Part model, mm, in its own coordinate system. Face numbers are marked on the shaded views. A direction names the side the tool comes from. Round coordinates to 2 decimals unless told otherwise and drop trailing zeros. Write each loop counter-clockwise with the first axis right and the second up, starting at its lowest first coordinate (ties: lowest second). Pieces come first, ordered by that corner, then holes. Notation, with made-up numbers: M 62,86 L 90,86 A22 ccw 90,105 Z; hole C 8,31 d8. An arc over 180 degrees is marked long. Use a Markdown table: item, result. Add a question column.
1) Slice it at D-D on x = 7.5. Write the cut outline in (y, z), plus the area to 3 significant figures.
2) Slice it at C-C on z = 10. Write the cut outline in (x, y), plus the area to 3 significant figures.
3) Slice it at B-B on y = 4. Write the cut outline in (x, z), plus the area to 3 significant figures.
4) Two-plate mould, pull along X, no slides. Class the marked faces 1, 2, 3 and 4: released by +X, released by -X, zero draft, split by the parting line, or undercut.
5) Which spindle directions (+Z, -Z, +X, -X, +Y, -Y) get a long thin tool onto all of the face, cutting with end or side? Do the marked faces 5 and 6. Say none if no direction does.
6) Slice it at A-A on x = 3.5. Write the cut outline in (y, z), plus the area to 3 significant figures.
7) Wall check: probe 1 along Z at (x, y) = (11.5, 6.25); probe 2 along X at (y, z) = (3.75, 9.25); probe 3 along Z at (x, y) = (7.25, 5). Give the ranges that are in metal, low to high.
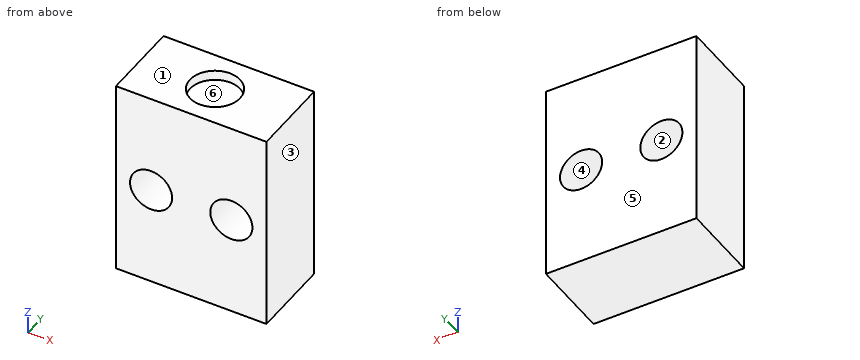
```python
from build123d import *

# Parameters (mm, degrees)
F0_W     = 15
F0_H     = 8
F1_DEPTH = 20
F2_R     = 2.1
F3_DEPTH = 25
F4_R     = 2.5
F5_DEPTH = 1


with BuildPart() as f1:
    # F0 (on Top) → F1 (new body)
    with BuildSketch(Plane.XY):
        with Locations((7.5, 4)):
            Rectangle(F0_W, F0_H)
    extrude(amount=F1_DEPTH)

    # F2 (on face) → F3 (cut)
    with BuildSketch(Plane.XZ):
        with Locations((3.5, 10)):
            Circle(F2_R)
        with Locations((11.5, 10)):
            Circle(F2_R)
    extrude(amount=-F3_DEPTH, mode=Mode.SUBTRACT)

    # F4 (on face) → F5 (cut)
    with BuildSketch(Plane.XY.offset(20)):
        with Locations((7.5, 4)):
            Circle(F4_R)
    extrude(amount=-F5_DEPTH, mode=Mode.SUBTRACT)


solid = f1.part
```
Entries:
| question | item | result |
|---|---|---|
| 1 | outline | M 0,0 L 8,0 L 8,20 L 6.5,20 L 6.5,19 L 1.5,19 L 1.5,20 L 0,20 Z |
| 1 | area | 155 mm^2 |
| 2 | outline | M 0,0 L 1.4,0 L 1.4,8 L 0,8 Z; M 5.6,0 L 9.4,0 L 9.4,8 L 5.6,8 Z; M 13.6,0 L 15,0 L 15,8 L 13.6,8 Z |
| 2 | area | 52.8 mm^2 |
| 3 | outline | M 0,0 L 15,0 L 15,20 L 10,20 L 10,19 L 5,19 L 5,20 L 0,20 Z; hole C 3.5,10 d4.2; hole C 11.5,10 d4.2 |
| 3 | area | 267 mm^2 |
| 4 | face 1 | zero draft |
| 4 | face 2 | undercut |
| 4 | face 3 | released by +X |
| 4 | face 4 | undercut |
| 5 | face 5 | +Z, -Z, +X, -X, +Y |
| 5 | face 6 | +Z |
| 6 | outline | M 0,0 L 8,0 L 8,7.9 L 0,7.9 Z; M 0,12.1 L 8,12.1 L 8,20 L 0,20 Z |
| 6 | area | 126 mm^2 |
| 7 | probe 1 | z = 0 to 7.9, 12.1 to 20 |
| 7 | probe 2 | x = 0 to 1.54, 5.46 to 9.54, 13.46 to 15 |
| 7 | probe 3 | z = 0 to 19 |
